from build123d import *

# Parameters (mm, degrees)
SKETCH1_W           = 21
SKETCH1_H           = 15
BOSS_EXTRUDE1_DEPTH = 2
BOSS_EXTRUDE2_DEPTH = 5
SKETCH3_W           = 19
SKETCH3_H           = 13
BOSS_EXTRUDE3_DEPTH = 11.8
SKETCH4_W           = 0.8
SKETCH4_H           = 4.8
BOSS_EXTRUDE4_DEPTH = 7.1
FILLET1_R           = 1.5875


with BuildPart() as part:
    # Sketch1 → Boss-Extrude1 (new body)
    with BuildSketch(Plane.XY):
        with Locations((10.5, 7.5)):
            Rectangle(SKETCH1_W, SKETCH1_H)
    extrude(amount=BOSS_EXTRUDE1_DEPTH)

    # Sketch2 → Boss-Extrude2 (add, symmetric)
    with BuildSketch(Plane(origin=(0, 7.5, 0), x_dir=(-1, 0, 0), z_dir=(0, -1, 0))):
        with BuildLine():
            Line((-14.818, 0), (-17.358, 0))
            add(Edge.make_bspline(
                [(-17.358, 0), (-16.707682386, 1.839588495), (-14.818, 3.5)],
                knots=[0, 0, 0, 1, 1, 1], degree=2))
            add(Edge.make_bspline(
                [(-14.818, 3.5), (-12.312840272, 1.371089101), (-7.964569246, 0.392132644), (-3.642, 0)],
                knots=[0, 0, 0, 0, 1, 1, 1, 1], degree=3))
            Line((-3.642, 0), (-14.818, 0))
        make_face()
    extrude(amount=BOSS_EXTRUDE2_DEPTH, both=True)

    # Sketch3 → Boss-Extrude3 (add)
    with BuildSketch(Plane.XY.offset(2)):
        with Locations((10.5, 7.5)):
            Rectangle(SKETCH3_W, SKETCH3_H)
    extrude(amount=BOSS_EXTRUDE3_DEPTH)

    # Sketch4 → Boss-Extrude4 (add)
    with BuildSketch(Plane.XY.offset(13.8)):
        with Locations((3.4, 7.5)):
            Rectangle(SKETCH4_W, SKETCH4_H)
        with Locations((10.5, 7.5)):
            Rectangle(SKETCH4_W, SKETCH4_H)
    extrude(amount=BOSS_EXTRUDE4_DEPTH)

    # Fillet1
    fillet1_edges = [part.edges().sort_by_distance(p)[0] for p in [
        (3.4, 5.1, 20.9),
        (3.4, 9.9, 20.9),
        (10.5, 5.1, 20.9),
        (10.5, 9.9, 20.9),
    ]]
    fillet(fillet1_edges, radius=FILLET1_R)


solid = part.part
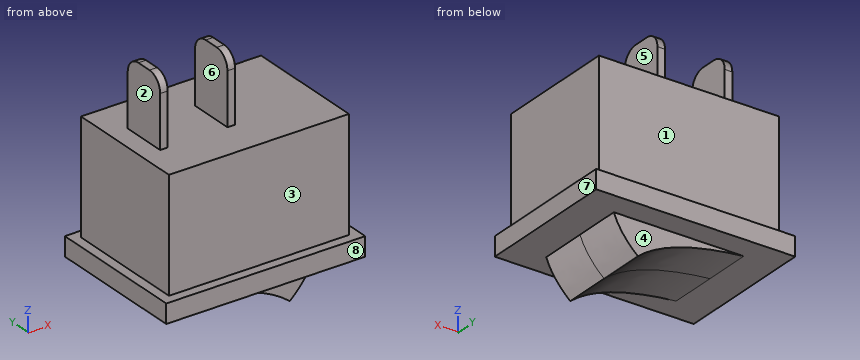
Could you check a few things on this model? Use its own coordinates, in mm. Face numbers are marked on the shaded views. A direction names the side the tool comes from. Round coordinates to 2 decimals unless told otherwise and drop trailing zeros. Write each loop counter-clockwise with the first axis right and the second up, starting at its lowest first coordinate (ties: lowest second). Pieces come first, ordered by that corner, then holes. Notation, with made-up numbers: (44, 64.5) -> (76, 64.5) arc R26 cw to (76, 85.5) -> close; hole circle Ø8 at (-33.75, 72). An arc over 180 degrees is marked (long way). Use a Markdown table: item, result.
1. If we section it at C-C (z = 9.75): List the corners of the cut face in (x, y) for me.
Answer key:
| item | result |
|---|---|
| outline | (1, 1) -> (20, 1) -> (20, 14) -> (1, 14) -> close |
2. We'd pull the mould along X, two halves only. Please class the marked faces 6, 7 and 8: +X half, -X half, draft (parallel to the pull), parting line (faces both ways), or undercut.
Answer key:
| item | result |
|---|---|
| face 6 | undercut |
| face 7 | +X half |
| face 8 | draft |
3. Which directions (+Z, -Z, +X, -X, +Y, -Y) give clear straight access to the entire face, cutting with the end or side of a thin tool? Please do the marked faces 1, 2, 3, 4 and 5.
Answer key:
| item | result |
|---|---|
| face 1 | +Z, +X, -X, +Y |
| face 2 | +Z, -X, +Y, -Y |
| face 3 | +Z, +X, -X, -Y |
| face 4 | -Z, +X, -X, +Y |
| face 5 | +Z, +X, +Y, -Y |
4. If we section it at B-B (x = 19.25): List the corners of the cut face in (y, z) for me.
Answer key:
| item | result |
|---|---|
| outline | (0, 0) -> (15, 0) -> (15, 2) -> (14, 2) -> (14, 13.8) -> (1, 13.8) -> (1, 2) -> (0, 2) -> close |
5. Please list where these lines run through material, in increasing order: probe 1 along Y at (x, z) = (2.75, 8.5); probe 2 along Z at (x, y) = (2.5, 9.5); probe 3 along X at (y, z) = (8, 17.5).
Answer key:
| item | result |
|---|---|
| probe 1 | y = 1 to 14 |
| probe 2 | z = 0 to 13.8 |
| probe 3 | x = 3 to 3.8, 10.1 to 10.9 |
6. If we section it at A-A (z = 17.5): List the corners of the cut face in (x, y) for me, then the cut area to 3 significant figures.
Answer key:
| item | result |
|---|---|
| outline | (3, 5.1) -> (3.8, 5.1) -> (3.8, 9.9) -> (3, 9.9) -> close; (10.1, 5.1) -> (10.9, 5.1) -> (10.9, 9.9) -> (10.1, 9.9) -> close |
| area | 7.68 mm^2 |
7. For pin 1 Ø5.5 at (y, z) = (7, 17) entering from +X; pin 2 Ø6 at (x, z) = (6, 9) entering from +Y; pin 3 Ø3.5 at (x, z) = (9, 5.5) entering from -Y, each with a flat end and sliding along its axis, tell me the tip position at first contact or that it passes through.
Answer key:
| item | result |
|---|---|
| pin 1 | stops at x = 10.9 |
| pin 2 | stops at y = 14 |
| pin 3 | stops at y = 1 |
